Source: CAD feature listing. Evaluate the final solid. Frame: model axes, mm. Face numbers are marked on the shaded views. A direction names the side the tool comes from. Give positions to 0.01 mm unless a question says otherwise; leave off trailing zeros. Write each loop counter-clockwise with the first axis right and the second up, starting at its lowest first coordinate (ties: lowest second). Pieces come first, ordered by that corner, then holes.
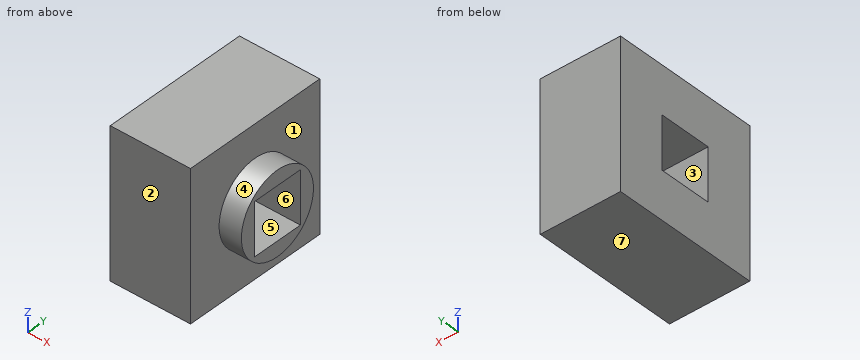
```python
from build123d import *

# Parameters (mm, degrees)
SKETCH2_W           = 23.3
SKETCH2_H           = 23.3
SKETCH2_W_2         = 8.3
SKETCH2_H_2         = 8.3
EXTRUDE_THIN1_DEPTH = 12.7
SKETCH3_R           = 6.5
SKETCH3_W           = 8.3
SKETCH3_H           = 8.3
BOSS_EXTRUDE1_DEPTH = 3.525


with BuildPart() as part:
    # Sketch2 → Extrude-Thin1 (new body)
    with BuildSketch(Plane(origin=(0, 0, 0), x_dir=(0, 0, -1), z_dir=(1, 0, 0))):
        with Locations((4.15, 4.15)):
            Rectangle(SKETCH2_W, SKETCH2_H)
        with Locations((4.15, 4.15)):
            Rectangle(SKETCH2_W_2, SKETCH2_H_2, mode=Mode.SUBTRACT)
    extrude(amount=EXTRUDE_THIN1_DEPTH)

    # Sketch3 → Boss-Extrude1 (add)
    with BuildSketch(Plane(origin=(12.7, 0, 0), x_dir=(0, 0, -1), z_dir=(1, 0, 0))):
        with Locations((4.15, 4.15)):
            Circle(SKETCH3_R)
        with Locations((4.15, 4.15)):
            Rectangle(SKETCH3_W, SKETCH3_H, mode=Mode.SUBTRACT)
    extrude(amount=BOSS_EXTRUDE1_DEPTH)


solid = part.part
```
1. Cut plane A-A, the plane z = -4.15. Return the cut outline in (x, y) (3 decimals).
2. Cut plane B-B, the plane y = 4.15. Return the cut outline in (x, z) (3 decimals), then the cut area to 3 significant figures.
3. Cut plane D-D, the plane z = -10. Return the cut outline in (x, y) (3 decimals).
4. Cut plane C-C, the plane x = 2.75. Return the cut outline in (y, z).
5. Access query for the marked faces 1, 2 and 3. Directions: +Z, -Z, +X, -X, +Y, -Y. A direction counts if a zero-diameter tool reaches every point of the face in a straight line with its end or side. Return the directions, or none.
6. Mould query, pull axis Y, two halves, no side actions, for the marked faces 4, 5, 6 and 7. Classes: +Y half, -Y half, draft (parallel to the pull), parting line (faces both ways), or undercut.
7. Line query: L1, parallel to Y at x = 3.75, z = -1.75; L2, parallel to Z at x = 3, y = 5.75; L3, parallel to X at y = 11.5, z = -11.5. Output: solid intervals per line, ascending.
Response values:
1. outline: (0, -7.5) - (12.7, -7.5) - (12.7, -2.35) - (16.225, -2.35) - (16.225, 0) - (0, 0) - close; (0, 8.3) - (16.225, 8.3) - (16.225, 10.65) - (12.7, 10.65) - (12.7, 15.8) - (0, 15.8) - close
2. outline: (0, -15.8) - (12.7, -15.8) - (12.7, -10.65) - (16.225, -10.65) - (16.225, -8.3) - (0, -8.3) - close; (0, 0) - (16.225, 0) - (16.225, 2.35) - (12.7, 2.35) - (12.7, 7.5) - (0, 7.5) - close
2. area: 207 mm2
3. outline: (0, -7.5) - (12.7, -7.5) - (12.7, 1.317) - (16.225, 1.317) - (16.225, 6.983) - (12.7, 6.983) - (12.7, 15.8) - (0, 15.8) - close
4. outline: (-7.5, -15.8) - (15.8, -15.8) - (15.8, 7.5) - (-7.5, 7.5) - close; hole (0, -8.3) - (8.3, -8.3) - (8.3, 0) - (0, 0) - close
5. face 1: +X
5. face 2: +Z, -Z, +X, -X, -Y
5. face 3: +X, -X
6. face 4: parting line
6. face 5: undercut
6. face 6: undercut
6. face 7: draft
7. L1: y = -7.5 to 0, 8.3 to 15.8
7. L2: z = -15.8 to -8.3, 0 to 7.5
7. L3: x = 0 to 12.7
